Autodesk Inventor part; units mm, degrees
ref_plane "YZ Plane" through (0, 0, 0) normal (1, 0, 0) x (0, 1, 0)
ref_plane "XZ Plane" through (0, 0, 0) normal (0, 1, 0) x (-1, 0, 0)
ref_plane "XY Plane" through (0, 0, 0) normal (0, 0, 1) x (1, 0, 0)
sketch "Main Sketch" plane through (0, 0, 0) normal (0, 1, 0) x (-1, 0, 0)
  line L0 (-57.375, -12.0472) -> (-57.375, 12.0472)
  line L1 (-57.375, 12.0472) -> (47.625, -10) construction
  line L2 (47.625, 10) -> (-57.375, -12.0472) construction
  circle A0 centre (47.625, 0) radius 7
  arc A1 (47.625, -10) -> (47.625, 10) centre (47.625, 0) ccw
  line L3 (-40.875, 17.5) -> (-57.375, 17.5)
  line L4 (-57.375, 17.5) -> (-57.375, -17.5)
  line L5 (-57.375, -17.5) -> (-40.875, -17.5)
  line L6 (-40.875, 17.5) -> (-57.375, -17.5) construction
  line L7 (-57.375, 17.5) -> (-40.875, -17.5) construction
  line L8 (47.625, -10) -> (-40.875, -10)
  line L9 (-40.875, -17.5) -> (-40.875, -10)
  line L10 (-40.875, 10) -> (-40.875, 17.5)
  line L11 (-40.875, 10) -> (47.625, 10)
  point P0 (0, 0)
  point P1 (-49.125, 0)
  dimension "d3" = 14
  dimension "d4" = 105
  dimension "d13" = 16.5
  dimension "d14" = 35
  dimension "d15" = 0
  dimension "d18" = 20
extrude "Main Extrusion" add sketch "Main Sketch" along normal blind 4
sketch "Screw Holes Sketch" plane through (0, 4, 0) normal (0, 1, 0) x (1, 0, 0)
  circle A0 centre (46.125, -8.75) radius 2
  line L0 (57.375, 17.5) -> (40.875, 17.5)
  line L1 (40.875, -17.5) -> (57.375, -17.5)
  line L2 (35.2664, 0) -> (65.7891, 0)
  line L3 (51.375, -27.0398) -> (51.375, 30.2346) construction
  line L4 (57.375, -17.5) -> (57.375, 17.5)
  line L5 (40.875, -10) -> (40.875, -17.5)
  circle A1 centre (46.125, 8.75) radius 2
  line L6 (51.375, 27.0398) -> (51.375, -30.2346) construction
  point P0 (0, 0)
  dimension "d21" = 4
  dimension "d22" = 35
  dimension "d23" = 6
  dimension "d24" = 5.25
  dimension "d25" = 5.25
  dimension "d26" = 10.5
  dimension "d27" = 8.75
  dimension "d28" = 17.5
extrude "Screw Holes Cut" cut sketch "Screw Holes Sketch" against normal through all
fillet "Smoooooooooooooooooth" radius 6 2 edges at (40.875, 2, -17.5) (40.875, 2, 17.5)
sketch "Side Axel Hole Sketch" plane through (-47.625, 0, 10) normal (0, 0, 1) x (1, 0, 0)
  line L0 (88.5, 4) -> (88.5, 0)
  line L1 (0, 0) -> (0, 4)
  line L2 (44.25, -12.0383) -> (44.25, 22.7681) construction
  line L3 (88.5, 0) -> (0, 0)
  line L4 (0, 4) -> (88.5, 4)
  circle A0 centre (44.25, 4) radius 1.5
  point P0 (47.625, 0)
  dimension "d32" = 88.5
  dimension "d33" = 44.25
  dimension "d34" = 44.25
  dimension "d35" = 4
  dimension "d41" = 3
extrude "Side Axel Hole Cut" cut sketch "Side Axel Hole Sketch" against normal blind 20 contours A0 L4 | L4 A0
sketch "Sketch6" plane through (-47.625, 0, 10) normal (0, 0, 1) x (1, 0, 0)
  arc A0 (42.75, 4) -> (45.75, 4) centre (44.25, 4) ccw
  circle A1 centre (44.25, 4) radius 3
  circle A2 centre (44.25, 4) radius 1.5
  point P0 (47.625, 0)
  dimension "d44" = 6
extrude "Extrusion7" add sketch "Sketch6" against normal blind 20
properties part number "TapeMeasureBracketSide"
Could you check a few things on this model? Use its own coordinates, in mm. A direction names the side the tool comes from. Give positions to 0.01 mm unless a question says otherwise; leave off trailing zeros. Order: outer loops, then holes, each group sorted by start corner. A loop starts at its lowest first (then second) coordinate and runs counter-clockwise, first axis right, second up. Notation, with made-up numbers: (-17.75, -33.75) -> (3.25, -33.75) arc R17 cw to (3.25, -21.75) -> close; hole circle Ø8 at (39, 79). An arc over 180 degrees is marked (long way). Answer in a Markdown table with one row per item. Add a question column.
Item 1: We'd pull the mould along X, two halves only. Please class faces 1 (the cylindrical face through (42.59, 2.03, 15.7)), 2 (the cylindrical face through (-3.3, 7, 0.1)), 3 (the flat face through (-4, 2, -10)), 4 (the cylindrical face through (-54.302, 1.972, -2.103)): pulls with the +X half, pulls with the -X half, needs draft (parallel to the pull), parting line crosses it, or undercut.
Item 2: Imagine slicing it at D-D (x = -27). List the corners of the cut face in (y, z) for me.
Item 3: I'm going to push flat-ended pins straight in: P1, Ø6, axis at x = -19, z = -4, coming from the +Y side; P2, Ø1, axis at y = 5, z = 8.5, coming from the +X side; P3, Ø1, axis at y = 4, z = -3, coming from the -X side; P4, Ø8.5, axis at x = -47.625, z = 0, coming from the -Y side. Where does each tip first touch, or does it pass through?
Item 4: Imagine slicing it at A-A (z = 0). List the corners of the cut face in (x, y) for me (3 decimals), and give its area (3 significant figures).
Item 5: For faces 5 (the flat face through (-26, 4, 0)), 6 (the flat face through (-4, 2, 10)), 7 (the flat face through (35, 4, 0)), 8 (the cylindrical face through (44.65, 2.03, -10.1)), which set-ups out of +Z, -Z, +X, -X, +Y, -Y let a thin tool reach every point of the face, with its end or its side?
Item 6: Please list where these lines run through material, in increasing order: probe 1 along X at (y, z) = (3.75, 0.5) (1 decimal); probe 2 along X at (y, z) = (4.25, 2); probe 3 along X at (y, z) = (3.5, -5.5) (3 decimals).
Item 7: Imagine slicing it at C-C (z = -8.75). List the corners of the cut face in (x, y) for me (3 decimals), and give its area (3 significant figures).
Item 8: Imagine slicing it at B-B (x = -43.5). List the corners of the cut face in (y, z) for me.
Result:
| question | item | result |
|---|---|---|
| 1 | face 1 | pulls with the -X half |
| 1 | face 2 | parting line crosses it |
| 1 | face 3 | needs draft |
| 1 | face 4 | undercut |
| 2 | outline | (0, -10) -> (4, -10) -> (4, 10) -> (0, 10) -> close |
| 3 | P1 | y = 4 |
| 3 | P2 | x = -0.42 |
| 3 | P3 | x = -57.31 |
| 3 | P4 | through |
| 4 | outline | (-57.625, 0) -> (-54.625, 0) -> (-54.625, 4) -> (-57.625, 4) -> close; (-40.625, 0) -> (57.375, 0) -> (57.375, 4) -> (-0.375, 4) arc R3 ccw to (-6.375, 4) -> (-40.625, 4) -> close; hole circle Ø3 at (-3.375, 4) |
| 4 | area | 411 mm2 |
| 5 | face 5 | +Z, -Z, -X, +Y |
| 5 | face 6 | +Z, -X, +Y, -Y |
| 5 | face 7 | +Z, -Z, +X, +Y |
| 5 | face 8 | +Y, -Y |
| 6 | probe 1 | -57.6 to -54.6, -40.6 to -4.9, -1.9 to 57.4 |
| 6 | probe 2 | -6.36 to -4.85, -1.9 to -0.39 |
| 6 | probe 3 | -55.977 to -51.955, -43.295 to -4.789, -1.961 to 57.375 |
| 7 | outline | (-52.466, 0) -> (44.125, 0) -> (44.125, 4) -> (-0.375, 4) arc R3 ccw to (-6.375, 4) -> (-52.466, 4) -> close; (48.125, 0) -> (57.375, 0) -> (57.375, 4) -> (48.125, 4) -> close; hole circle Ø3 at (-3.375, 4) |
| 7 | area | 430 mm2 |
| 8 | outline | (0, -10) -> (4, -10) -> (4, -5.66) -> (0, -5.66) -> close; (0, 5.66) -> (4, 5.66) -> (4, 10) -> (0, 10) -> close |
